Geometry: see drawing. Coordinates: mm, zero at the bounding-box minimum. A direction names the side the tool comes from. Round coordinates to 2 decimals unless told otherwise and drop trailing zeros. Loops run counter-clockwise (first coordinate to the right, second up) from the corner with the lowest first, then second, coordinate; pieces in that order, holes last. Notation, with made-up numbers: (55.5, 6.25) - (102.5, 6.25) arc R20 cw to (102.5, 35.25) - close; hole circle Ø6 at (65, 76). An arc over 180 degrees is marked (long way). Return JSON: item names as keys, results as strings. Group by question number.
1. Material intervals for probe 1 along X at (y, z) = (13.5, 24); probe 2 along Z at (x, y) = (33, 11.5); probe 3 along Y at (x, z) = (24, 31), sorted ascending.
2. First-contact query: pin 1 Ø6 at (x, y) = (34, 10.5) entering from -Z; pin 2 Ø8 at (x, y) = (44.5, 44) entering from +Z; pin 3 Ø1.5 at (x, y) = (22, 23.5) entering from +Z. Flat tips, straight axial feed; report the tip coordinate or a pass-through.
3. Set-up query: the marked faces 1 and 2. Return all of +Z, -Z, +X, -X, +Y, -Y with unobstructed straight access to the full face (end or side cutting, diameter ignored); none if empty.
4. Section B-B on x = 15.5. Return loops of the section in (y, z).
5. Section C-C on z = 22.5. Return loops of the section in (x, y).
6. Section D-D on y = 8.5. Return loops of the section in (x, z).
7. Section A-A on y = 34.5. Return loops of the section in (x, z), and give its area (3 significant figures).
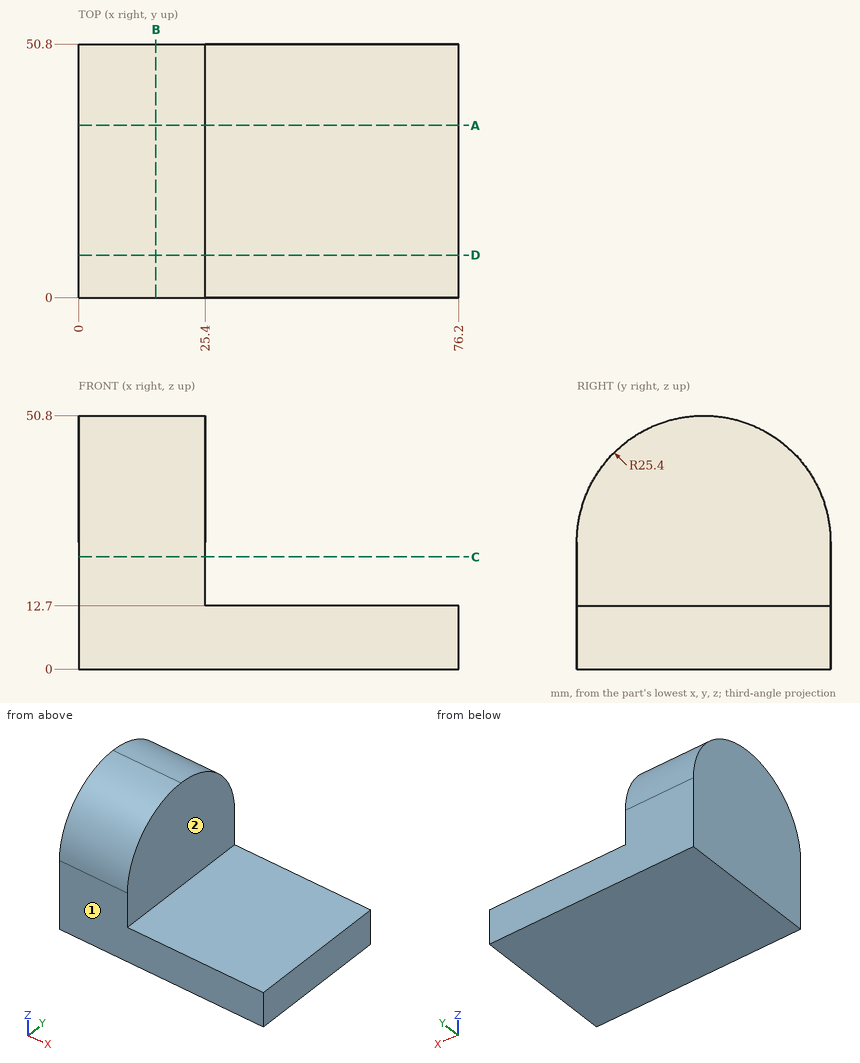
Taken from the geometry:
{
 "1": {"probe 1": "0 to 25.4", "probe 2": "0 to 12.7", "probe 3": "0.63 to 50.17"},
 "2": {"pin 1": "z = 0", "pin 2": "z = 12.7", "pin 3": "z = 50.77"},
 "3": {"face 1": "+Z, -Z, +X, -X, -Y", "face 2": "+Z, +X, +Y, -Y"},
 "4": {"outline": "(0, 0) - (50.8, 0) - (50.8, 25.4) arc R25.4 ccw to (25.4, 50.8) arc R25.4 ccw to (0, 25.4) - close"},
 "5": {"outline": "(0, 0) - (25.4, 0) - (25.4, 50.8) - (0, 50.8) - close"},
 "6": {"outline": "(0, 0) - (76.2, 0) - (76.2, 12.7) - (25.4, 12.7) - (25.4, 44.36) - (0, 44.36) - close"},
 "7": {"outline": "(0, 0) - (76.2, 0) - (76.2, 12.7) - (25.4, 12.7) - (25.4, 49.11) - (0, 49.11) - close", "area": "1,890 mm2"}
}
